Geometry check sheet. Reference: the model listing, model coordinates, mm. A direction names the side the tool comes from. Give positions to 0.01 mm unless a question says otherwise; leave off trailing zeros. Loops run counter-clockwise (first coordinate to the right, second up) from the corner with the lowest first, then second, coordinate; pieces in that order, holes last. Notation, with made-up numbers: (-35.5, 58.25) -> (-24.5, 58.25) arc R19 ccw to (-24.5, 91.25) -> close; hole circle Ø2 at (16, -7.75). An arc over 180 degrees is marked (long way). Write each question's results on one line, items separated by ' | '. Start each with the question number.
1) Set-up check for faces 5 (the face through (0, -4, 25)), 6 (the face through (28, -4, 10)), 7 (the face through (62.5, -4, 61)), 8 (the face through (-106, -4, 28)): record each of +Z, -Z, +X, -X, +Y, -Y from which the full face is reachable in a straight line by a thin tool's end or side.
2) Sectioned sample at C-C on z = 9.5. Record the cut outline in (x, y), then the cut area to 3 significant figures.
3) Sectioned sample at B-B on y = -6.75. Record the cut outline in (x, z), then the cut area to 3 significant figures.
4) Sectioned sample at A-A on x = -23.5. Record the cut outline in (y, z), then the cut area to 3 significant figures.
5) Depth check by flat-ended pin: pin 1 (4 mm diameter, centred on y = -3.5, z = 31.5, fed in from -X); pin 2 (4 mm diameter, centred on x = 97, y = -3.5, fed in from +Z); pin 3 (4 mm diameter, centred on x = 9.5, y = -4, fed in from -Z). Enter the tip coordinate at first touch or a pass-through.
6) Sectioned sample at D-D on z = 65. Record the cut outline in (x, y), then the cut area to 3 significant figures.
7) Scan lines: line 1 (X direction, y = -2, z = 35); line 2 (Z direction, x = -12, y = -4); line 3 (X direction, y = -0.5, z = 17). Record each from-to range of solid material in increasing order. Write a range as from..to.
8) Draft check along Z on faces 1 (the face through (0, -4, 20)), 2 (the face through (-28, -4, 10)), 3 (the face through (0, -4, 45)), 4 (the face through (28, -4, 35)). Enter one of: pulls with the +Z half, pulls with the -Z half, needs draft (parallel to the pull), parting line crosses it, or undercut.
```python
from build123d import *

# Parameters (mm, degrees)
F1_DEPTH = 8
F2_W     = 56
F2_H     = 20
F3_DEPTH = 25
F5_W     = 28
F5_H     = 20
F6_DEPTH = 25


with BuildPart() as f1:
    # F0 (on Front) → F1 (new body)
    with BuildSketch(Plane.XZ):
        Polygon((-150, 0), (0, 0), (150, 0), (150, 28), (62.5, 28), (62.5, 95), (-62.5, 95), (-62.5, 28), (-150, 28), align=None)
    extrude(amount=F1_DEPTH)

    # F2 (on face) → F3 (cut)
    with BuildSketch(Plane.XZ.offset(8)):
        with Locations((0, 10)):
            Rectangle(F2_W, F2_H)
    extrude(amount=-F3_DEPTH, mode=Mode.SUBTRACT)

    # F5 (on face) → F6 (cut)
    with BuildSketch(Plane.XZ.offset(8)):
        with Locations((-14, 35)):
            Rectangle(F5_W, F5_H)
        with Locations((14, 35)):
            Rectangle(F5_W, F5_H)
    extrude(amount=-F6_DEPTH, mode=Mode.SUBTRACT)


solid = f1.part
```
Result:
1) face 5: +Y, -Y | face 6: -Z, +Y, -Y | face 7: +Z, +X, +Y, -Y | face 8: +Z, -X, +Y, -Y
2) outline: (-150, -8) -> (-28, -8) -> (-28, 0) -> (-150, 0) -> close; (28, -8) -> (150, -8) -> (150, 0) -> (28, 0) -> close | area: 1,950 mm^2
3) outline: (-150, 0) -> (-28, 0) -> (-28, 20) -> (28, 20) -> (28, 0) -> (150, 0) -> (150, 28) -> (62.5, 28) -> (62.5, 95) -> (-62.5, 95) -> (-62.5, 28) -> (-150, 28) -> close; hole (-28, 25) -> (28, 25) -> (28, 45) -> (-28, 45) -> close | area: 14,500 mm^2
4) outline: (-8, 20) -> (0, 20) -> (0, 25) -> (-8, 25) -> close; (-8, 45) -> (0, 45) -> (0, 95) -> (-8, 95) -> close | area: 440 mm^2
5) pin 1: x = -62.5 | pin 2: z = 28 | pin 3: z = 20
6) outline: (-62.5, -8) -> (62.5, -8) -> (62.5, 0) -> (-62.5, 0) -> close | area: 1,000 mm^2
7) line 1: -62.5..-28, 28..62.5 | line 2: 20..25, 45..95 | line 3: -150..-28, 28..150
8) face 1: pulls with the -Z half | face 2: needs draft | face 3: undercut | face 4: undercut
